from build123d import *

# Parameters (mm, degrees)
SKETCH1_R           = 14
SKETCH1_W           = 18
SKETCH1_H           = 38
BOSS_EXTRUDE1_DEPTH = 15
FILLET1_R           = 40


with BuildPart() as part:
    # Sketch1 → Boss-Extrude1 (new body)
    with BuildSketch(Plane.XY):
        Polygon((186.455659815, 80), (-186.455659815, 80), (0, -48.590110217), align=None)
        Circle(SKETCH1_R, mode=Mode.SUBTRACT)
        with Locations((-58, 40)):
            Rectangle(SKETCH1_W, SKETCH1_H, mode=Mode.SUBTRACT)
        with Locations((58, 40)):
            Rectangle(SKETCH1_W, SKETCH1_H, mode=Mode.SUBTRACT)
    extrude(amount=BOSS_EXTRUDE1_DEPTH)

    # Fillet1
    fillet1_edges = [part.edges().sort_by_distance(p)[0] for p in [
        (0, -48.590110217, 7.5),
        (-186.455659815, 80, 7.5),
        (186.455659815, 80, 7.5),
    ]]
    fillet(fillet1_edges, radius=FILLET1_R)


solid = part.part
The listing builds one solid part. Answer for the finished solid, in the listing's coordinates (mm). A direction names the side the tool comes from. Coordinates: 2 decimals unless noted, no trailing zeros. Write each loop counter-clockwise with the first axis right and the second up, starting at its lowest first coordinate (ties: lowest second). Pieces come first, ordered by that corner, then holes. Notation, with made-up numbers: M 82,50.25 L 96,50.25 A29 ccw 96,79.25 Z; hole C 31,-38 d3. An arc over 180 degrees is marked long. Use one line per item in the form item = value.
Item 1: Find the intervals of material crossed by probe 1 along Y at (x, z) = (0, 7); probe 2 along X at (y, z) = (54, 13.5); probe 3 along X at (y, z) = (28, 4.5), in increasing order.
Model answer:
probe_1 = -40 to -14, 14 to 80
probe_2 = -95.47 to -67, -49 to 49, 67 to 95.47
probe_3 = -96.16 to -67, -49 to 49, 67 to 96.16
Item 2: Find section C-C, the plane y = 26. Give the vertices of the cut face in (x, z), plus the area to 3 significant figures.
Model answer:
outline = M -95.47,0 L -67,0 L -67,15 L -95.47,15 Z; M -49,0 L 49,0 L 49,15 L -49,15 Z; M 67,0 L 95.47,0 L 95.47,15 L 67,15 Z
area = 2,320 mm2
Item 3: Find section D-D, the plane y = 0. Give the vertices of the cut face in (x, z), plus the area to 3 significant figures.
Model answer:
outline = M -70.46,0 L -14,0 L -14,15 L -70.46,15 Z; M 14,0 L 70.46,0 L 70.46,15 L 14,15 Z
area = 1,690 mm2
Item 4: Given P1, Ø4.5, axis at y = 48, z = 9.5, coming from the +X side; P2, Ø5, axis at y = -22.5, z = 3, coming from the +X side; P3, Ø4.5, axis at x = 61.5, z = 5, coming from the +Y side, each flat-ended and moving along its own axis, determine where each tip first touches the part or whether it passes through.
Model answer:
P1 = 97.58
P2 = 41.46
P3 = 79.98
Item 5: The mould has two halves that part along X. Classify faces 3 (the face through (-52.115, -12.649, 7.395)), 4 (the face through (0, -40, 8)), 5 (the face through (58, 59, 7)): released by +X, released by -X, zero draft, split by the parting line, or undercut.
Model answer:
face_3 = released by -X
face_4 = split by the parting line
face_5 = undercut
Item 6: Find section A-A, the plane x = 0. Give the vertices of the cut face in (y, z).
Model answer:
outline = M -40,0 L -14,0 L -14,15 L -40,15 Z; M 14,0 L 80,0 L 80,15 L 14,15 Z
Item 7: Find section B-B, the plane z = 2. Give the vertices of the cut face in (x, y).
Model answer:
outline = M -80.71,7.07 L -22.71,-32.93 A40 ccw 22.71,-32.93 L 80.71,7.07 A40 ccw 58,80 L -58,80 A40 ccw Z; hole M -67,21 L -49,21 L -49,59 L -67,59 Z; hole C 0,0 d28; hole M 49,21 L 67,21 L 67,59 L 49,59 Z
Item 8: For faces 1 (the face through (95.974, 52.569, 7.605)), 2 (the face through (-58, 21, 7)), determine the directions among +Z, -Z, +X, -X, +Y, -Y from which every point of the face is accessible in a straight line to the end or side of a thin tool.
Model answer:
face_1 = +Z, -Z, +X
face_2 = +Z, -Z
